from build123d import *

# Parameters (mm, degrees)
F0_R     = 2.3876
F1_DEPTH = 3.81
F2_R     = 3.96875
F3_DEPTH = 5.08
F4_R     = 1.59385
F5_DEPTH = 2.921
F6_R     = 0.254


with BuildPart() as f1:
    # F0 (on Front) → F1 (new body)
    with BuildSketch(Plane.XZ):
        Circle(F0_R)
    extrude(amount=F1_DEPTH)

    # F2 (on face) → F3 (join)
    with BuildSketch(Plane.XZ.offset(3.81)):
        Circle(F2_R)
    extrude(amount=F3_DEPTH)

    # F4 (on face) → F5 (cut)
    with BuildSketch(Plane(origin=(0, 0, 0), x_dir=(-1, 0, 0), z_dir=(0, 1, 0))):
        Circle(F4_R)
    extrude(amount=-F5_DEPTH, mode=Mode.SUBTRACT)

    # F6
    f6_edges = [f1.edges().sort_by_distance(p)[0] for p in [
        (-3.96875, -3.81, 0),
    ]]
    fillet(f6_edges, radius=F6_R)


solid = f1.part
Read the model definition and answer for the solid it produces. Units are mm, in the model's axes. A direction names the side the tool comes from. Give positions to 0.01 mm unless a question says otherwise; leave off trailing zeros. Write each loop counter-clockwise with the first axis right and the second up, starting at its lowest first coordinate (ties: lowest second). Pieces come first, ordered by that corner, then holes. Notation, with made-up numbers: (-35.5, 9.25) -> (-16.5, 9.25) arc R36 ccw to (-16.5, 47.25) -> close; hole circle Ø5 at (-27.75, -7.5). An arc over 180 degrees is marked (long way). Answer as a JSON object with one key per item and string values. Group by question number.
1) Find section D-D (y = -6). Write down the section's boundary in (x, z).
2) Consider L1, parallel to Z at x = 0, y = -1.2; L2, parallel to Y at x = -3, z = -1.5; L3, parallel to Y at x = -0.75, z = -1. Determine where each line is inside the solid, lowest interval first. Write a range as from..to.
3) Find section C-C (y = -1.5). Write down the section's boundary in (x, z), and give its area (3 significant figures).
4) Each of these flat-tipped pins is pushed along its axis until it touches: P1, Ø1.5, axis at x = 0.5, y = -2, coming from the +Z side; P2, Ø1.5, axis at y = -7.5, z = -2.5, coming from the -X side; P3, Ø1, axis at y = -2.5, z = 3, coming from the -X side; P4, Ø1.6, axis at x = 0.5, z = 0.5, coming from the +Y side. Where does it stop, or does it pass through?
5) Find section A-A (z = 0). Write down the section's boundary in (x, y), and give its area (3 significant figures).
6) Find section B-B (x = 0). Write down the section's boundary in (y, z).
7) A tool of negligible diameter and unlimited length cuts with its end or side. For faces 1 (the flat face through (2.42, -3.81, -0.77)), 2 (the flat face through (0, -8.89, 0)), from which of +Z, -Z, +X, -X, +Y, -Y can it reach the whole face along a straight path? Write none if from no direction.
8) The mould has two halves that part along X. Classify faces 3 (the flat face through (0, -2.921, 0)), 4 (the cylindrical face through (-0.86, -6.443, -3.874)), 5 (the flat face through (2, 0, 0)): +X half, -X half, draft (parallel to the pull), parting line (faces both ways), or undercut.
Values follow:
{
 "1": {"outline": "circle Ø7.94 at (0, 0)"},
 "2": {"L1": "z = -2.39..-1.59, 1.59..2.39", "L2": "y = -8.89..-3.81", "L3": "y = -8.89..-2.92"},
 "3": {"outline": "circle Ø4.78 at (0, 0); hole circle Ø3.19 at (0, 0)", "area": "9.93 mm2"},
 "4": {"P1": "stops at z = 2.39", "P2": "stops at x = -3.56", "P3": "passes through", "P4": "stops at y = -2.92"},
 "5": {"outline": "(-3.97, -8.89) -> (3.97, -8.89) -> (3.97, -4.06) arc R0.25 ccw to (3.71, -3.81) -> (2.39, -3.81) -> (2.39, 0) -> (1.59, 0) -> (1.59, -2.92) -> (-1.59, -2.92) -> (-1.59, 0) -> (-2.39, 0) -> (-2.39, -3.81) -> (-3.71, -3.81) arc R0.25 ccw to (-3.97, -4.06) -> close", "area": "49.2 mm2"},
 "6": {"outline": "(-8.89, -3.97) -> (-4.06, -3.97) arc R0.25 ccw to (-3.81, -3.71) -> (-3.81, -2.39) -> (0, -2.39) -> (0, -1.59) -> (-2.92, -1.59) -> (-2.92, 1.59) -> (0, 1.59) -> (0, 2.39) -> (-3.81, 2.39) -> (-3.81, 3.71) arc R0.25 ccw to (-4.06, 3.97) -> (-8.89, 3.97) -> close"},
 "7": {"face 1": "+Y", "face 2": "+Z, -Z, +X, -X, -Y"},
 "8": {"face 3": "undercut", "face 4": "parting line", "face 5": "draft"}
}
